The listing builds one solid part. Answer for the finished solid, in the listing's coordinates (mm). Face numbers are marked on the shaded views. A direction names the side the tool comes from. Round coordinates to 2 decimals unless told otherwise and drop trailing zeros. Write each loop counter-clockwise with the first axis right and the second up, starting at its lowest first coordinate (ties: lowest second). Pieces come first, ordered by that corner, then holes. Notation, with made-up numbers: (46.25, -40) - (96.25, -40) arc R20 ccw to (96.25, -30) - close; hole circle Ø9 at (49.25, 14.5). An arc over 180 degrees is marked (long way). Answer in a Markdown table with one row per item.
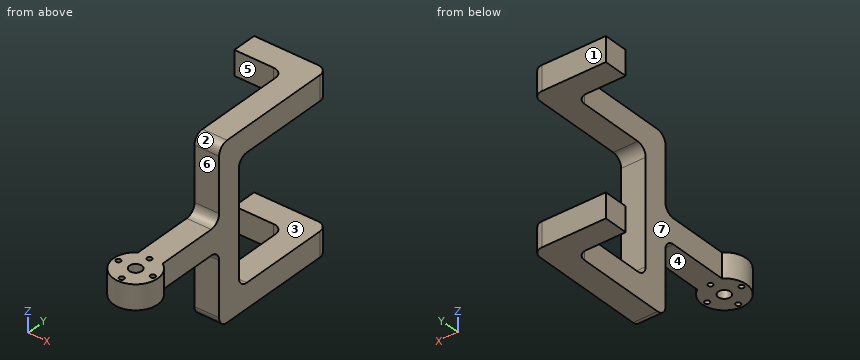
from build123d import *

# Parameters (mm, degrees)
ESQUISSE1_R        = 2.5
ESQUISSE1_R_2      = 1
BOSS_EXTRU_1_DEPTH = 10
BOSS_EXTRU_2_DEPTH = 10
ESQUISSE5_W        = 10
ESQUISSE5_H        = 10
BOSS_EXTRU_3_DEPTH = 20
CONG_1_R           = 4


with BuildPart() as part:
    # Esquisse1 → Boss.-Extru.1 (new body)
    with BuildSketch(Plane.XY):
        with BuildLine():
            Line((4, 55), (14, 55))
            Line((14, 55), (14, 16.483314774))
            ThreePointArc((14, 16.483314774), (9, 0), (4, 16.483314774))
            Line((4, 16.483314774), (4, 55))
        make_face()
        with Locations((9, 9)):
            Circle(ESQUISSE1_R, mode=Mode.SUBTRACT)
        with Locations((9, 16)):
            Circle(ESQUISSE1_R_2, mode=Mode.SUBTRACT)
        with Locations((16, 9)):
            Circle(ESQUISSE1_R_2, mode=Mode.SUBTRACT)
        with Locations((9, 2)):
            Circle(ESQUISSE1_R_2, mode=Mode.SUBTRACT)
        with Locations((2, 9)):
            Circle(ESQUISSE1_R_2, mode=Mode.SUBTRACT)
    extrude(amount=BOSS_EXTRU_1_DEPTH)

    # Esquisse4 → Boss.-Extru.2 (add)
    with BuildSketch(Plane(origin=(14, 0, 0), x_dir=(0, 0, -1), z_dir=(1, 0, 0))):
        Polygon((-30, 55), (20, 55), (20, 100), (30, 100), (30, 45), (-40, 45), (-40, 100), (-30, 100), align=None)
    extrude(amount=-BOSS_EXTRU_2_DEPTH)

    # Esquisse5 → Boss.-Extru.3 (add)
    with BuildSketch(Plane.ZY.offset(-4)):
        with Locations((-25, 95)):
            Rectangle(ESQUISSE5_W, ESQUISSE5_H)
        with Locations((35, 95)):
            Rectangle(ESQUISSE5_W, ESQUISSE5_H)
    extrude(amount=BOSS_EXTRU_3_DEPTH)

    # Congé1
    cong_1_edges = [part.edges().sort_by_distance(p)[0] for p in [
        (9, 45, 0),
        (9, 45, -30),
        (14, 100, -25),
        (9, 55, -20),
        (9, 45, 10),
        (9, 45, 40),
        (9, 55, 30),
        (14, 100, 35),
        (4, 90, -25),
        (4, 90, 35),
    ]]
    fillet(cong_1_edges, radius=CONG_1_R)


solid = part.part
(1) Section D-D (z = 33) is taken. Give the vertices of the cut face in (x, y).
Checked values:
| item | result |
|---|---|
| outline | (-16, 90) - (0, 90) arc R4 cw to (4, 86) - (4, 45) - (14, 45) - (14, 96) arc R4 ccw to (10, 100) - (-16, 100) - close |
(2) Find the intervals of material crossed by line 1 (Y direction, x = 9, z = 3); line 2 (X direction, y = 51.5, z = -0.5); line 3 (Z direction, x = 6, y = 81.5), in increasing order.
Checked values:
| item | result |
|---|---|
| line 1 | y = 0 to 1, 3 to 6.5, 11.5 to 15, 17 to 55 |
| line 2 | x = 4 to 14 |
| line 3 | z = -30 to -20, 30 to 40 |
(3) Section A-A (x = -13) is taken. Give the vertices of the cut face in (y, z).
Checked values:
| item | result |
|---|---|
| outline | (90, -30) - (100, -30) - (100, -20) - (90, -20) - close; (90, 30) - (100, 30) - (100, 40) - (90, 40) - close |
(4) Section B-B (y = 57) is taken. Give the vertices of the cut face in (x, z).
Checked values:
| item | result |
|---|---|
| outline | (4, -30) - (14, -30) - (14, -19.46) - (4, -19.46) - close; (4, 29.46) - (14, 29.46) - (14, 40) - (4, 40) - close |
(5) Section C-C (z = 3) is taken. Give the vertices of the cut face in (x, y).
Checked values:
| item | result |
|---|---|
| outline | (4, 16.48) arc R9 ccw (long way) to (14, 16.48) - (14, 55) - (4, 55) - close; hole circle Ø2 at (2, 9); hole circle Ø5 at (9, 9); hole circle Ø2 at (9, 2); hole circle Ø2 at (9, 16); hole circle Ø2 at (16, 9) |
(6) For a pull along Z with two mould halves and no side action, classify the marked faces 1, 2, 3 and 4 as pulls with the +Z half, pulls with the -Z half, needs draft (parallel to the pull), parting line crosses it, or undercut.
Checked values:
| item | result |
|---|---|
| face 1 | needs draft |
| face 2 | pulls with the +Z half |
| face 3 | undercut |
| face 4 | pulls with the -Z half |
(7) Flat-ended cylindrical pins translate along their axes: pin 1 (10 mm diameter, centred on y = 36.5, z = -2, fed in from +X); pin 2 (12 mm diameter, centred on x = 12, y = 26, fed in from +Z); pin 3 (5 mm diameter, centred on x = -11.5, z = 37.5, fed in from -Y); pin 4 (1.6 mm diameter, centred on x = 16, y = 9, fed in from +Z). Find the tip coordinate at first contact, or state that the pin passes through.
Checked values:
| item | result |
|---|---|
| pin 1 | stops at x = 14 |
| pin 2 | stops at z = 10 |
| pin 3 | stops at y = 90 |
| pin 4 | passes through |
(8) For the marked faces 5, 6 and 7, determine the directions among +Z, -Z, +X, -X, +Y, -Y from which every point of the face is accessible in a straight line to the end or side of a thin tool.
Checked values:
| item | result |
|---|---|
| face 5 | +Z, -Z, -X, -Y |
| face 6 | +Z, +X, -X, -Y |
| face 7 | +Z, -Z, -X |
